from build123d import *

# Parameters (mm, degrees)
SKETCH1_W           = 100
SKETCH1_H           = 400
SKETCH1_W_2         = 31
SKETCH1_H_2         = 354
BOSS_EXTRUDE1_DEPTH = 4
SKETCH2_W           = 20.5
SKETCH2_H           = 337
BOSS_EXTRUDE2_DEPTH = 4


with BuildPart() as part:
    # Sketch1 → Boss-Extrude1 (new body)
    with BuildSketch(Plane(origin=(0, 0, 0), x_dir=(0, 0, -1), z_dir=(1, 0, 0))):
        with Locations((0, 200)):
            Rectangle(SKETCH1_W, SKETCH1_H)
        with Locations((0, 200)):
            Rectangle(SKETCH1_W_2, SKETCH1_H_2, mode=Mode.SUBTRACT)
    extrude(amount=BOSS_EXTRUDE1_DEPTH)

    # Sketch2 → Boss-Extrude2 (add)
    with BuildSketch(Plane.ZY):
        with Locations((5.25, 208.5)):
            Rectangle(SKETCH2_W, SKETCH2_H)
    extrude(amount=-BOSS_EXTRUDE2_DEPTH)


solid = part.part
Work out the finished part from the listing and answer in its coordinate system (mm). Round coordinates to 2 decimals unless told otherwise and drop trailing zeros. Loops run counter-clockwise (first coordinate to the right, second up) from the corner with the lowest first, then second, coordinate; pieces in that order, holes last. Notation, with made-up numbers: (-33, 57) -> (-1, 57) arc R10 ccw to (-1, 68) -> close; hole circle Ø5 at (-36, 23). An arc over 180 degrees is marked (long way). Use one line per item in the form item = value.
(1) Find section C-C on z = 2.5. Give the vertices of the cut face in (x, y).
Answer list:
outline = (0, 0) -> (4, 0) -> (4, 23) -> (0, 23) -> close; (0, 40) -> (4, 40) -> (4, 400) -> (0, 400) -> close
(2) Find section B-B on y = 245. Give the vertices of the cut face in (x, z), then the cut area to 3 significant figures.
Answer list:
outline = (0, -50) -> (4, -50) -> (4, -15.5) -> (0, -15.5) -> close; (0, -5) -> (4, -5) -> (4, 50) -> (0, 50) -> close
area = 358 mm2
(3) Find section A-A on x = 3.1. Give the vertices of the cut face in (y, z), then the cut area to 3 significant figures.
Answer list:
outline = (0, -50) -> (400, -50) -> (400, 50) -> (0, 50) -> close; hole (23, -15.5) -> (377, -15.5) -> (377, -5) -> (40, -5) -> (40, 15.5) -> (23, 15.5) -> close
area = 35,900 mm2
(4) Straight lines are drawn through the part: line 1 (Y direction, x = 3.3, z = 4.5); line 2 (Z direction, x = 0.45, y = 216.5); line 3 (Y direction, x = 0.75, z = -11). For each, find the intervals that lie inside material, in ascending order.
Answer list:
line_1 = 0 to 23, 40 to 400
line_2 = -50 to -15.5, -5 to 50
line_3 = 0 to 23, 377 to 400
